from build123d import *

# Parameters (mm, degrees)
F0_W      = 120
F0_H      = 62
F1_DEPTH  = 1.5
F3_DEPTH  = 1.501
F5_DEPTH  = 1.501
F7_DEPTH  = 1.501
F8_R      = 1
F9_DEPTH  = 1.501
F10_W     = 7
F10_H     = 5
F11_DEPTH = 2
F13_DEPTH = 1
F14_W     = 3
F14_H     = 2.5
F15_DEPTH = 2
F16_W     = 3
F16_H     = 2.5
F17_DEPTH = 2
F18_W     = 3
F18_H     = 1
F19_DEPTH = 1
F20_W     = 4
F20_H     = 3
F21_DEPTH = 1
F23_DEPTH = 3
F24_W     = 1.5
F24_H     = 3
F25_DEPTH = 1
F26_W     = 5
F26_H     = 3.5
F27_DEPTH = 1.5
F28_W     = 3
F28_H     = 2
F29_DEPTH = 2
F30_W     = 3
F30_H     = 2
F31_DEPTH = 2
F32_R     = 2.5
F33_DEPTH = 2
F34_R     = 2.5
F35_DEPTH = 2
F36_W     = 3
F36_H     = 4
F37_DEPTH = 1
F38_W     = 2
F38_H     = 3
F39_DEPTH = 2


with BuildPart() as f1:
    # F0 (on Top) → F1 (new body)
    with BuildSketch(Plane.XY):
        with Locations((-17.615131, 6.410271)):
            Rectangle(F0_W, F0_H)
    extrude(amount=F1_DEPTH)

    # F2 (on face) → F3 (cut, through all)
    with BuildSketch(Plane.XY.offset(1.5)):
        with BuildLine():
            Line((-62.615131, -18.589729), (-62.615131, -24.589729))
            Line((-62.615131, -24.589729), (-34.615131, -24.589729))
            Line((-34.615131, -24.589729), (-34.615131, -18.589729))
            ThreePointArc((-34.615131, -18.589729), (-34.908024, -17.882622), (-35.615131, -17.589729))
            Line((-35.615131, -17.589729), (-61.615131, -17.589729))
            ThreePointArc((-61.615131, -17.589729), (-62.322238, -17.882622), (-62.615131, -18.589729))
        make_face()
    extrude(amount=-F3_DEPTH, mode=Mode.SUBTRACT)

    # F4 (on face) → F5 (cut, through all)
    with BuildSketch(Plane.XY.offset(1.5)):
        with BuildLine():
            Line((-20.615131, -17.589729), (-20.615131, -24.589729))
            Line((-20.615131, -24.589729), (-18.615131, -24.589729))
            Line((-18.615131, -24.589729), (-18.615131, -17.589729))
            ThreePointArc((-18.615131, -17.589729), (-19.615131, -16.589729), (-20.615131, -17.589729))
        make_face()
    extrude(amount=-F5_DEPTH, mode=Mode.SUBTRACT)

    # F6 (on face) → F7 (cut, through all)
    with BuildSketch(Plane.XY.offset(1.5)):
        with BuildLine():
            Line((22.384869, -17.543457), (22.384869, -24.589729))
            Line((22.384869, -24.589729), (24.384869, -24.589729))
            Line((24.384869, -24.589729), (24.384869, -17.543457))
            ThreePointArc((24.384869, -17.543457), (23.384869, -16.543457), (22.384869, -17.543457))
        make_face()
    extrude(amount=-F7_DEPTH, mode=Mode.SUBTRACT)

    # F8 (on face) → F9 (cut, through all)
    with BuildSketch(Plane.XY.offset(1.5)):
        with Locations((39.384869, -10.589729)):
            Circle(F8_R)
    extrude(amount=-F9_DEPTH, mode=Mode.SUBTRACT)

    # F10 (on face) → F11 (join)
    with BuildSketch(Plane.XY.offset(1.5)):
        with Locations((26.884869, -0.089729)):
            Rectangle(F10_W, F10_H)
    extrude(amount=F11_DEPTH)

    # F12 (on face) → F13 (join)
    with BuildSketch(Plane.XY.offset(1.5)):
        with BuildLine():
            Line((9.384869, 10.410271), (-2.615131, 10.410271))
            ThreePointArc((-2.615131, 10.410271), (-3.322238, 10.117378), (-3.615131, 9.410271))
            Line((-3.615131, 9.410271), (-3.615131, -8.589729))
            ThreePointArc((-3.615131, -8.589729), (-3.322238, -9.296836), (-2.615131, -9.589729))
            Line((-2.615131, -9.589729), (9.384869, -9.589729))
            ThreePointArc((9.384869, -9.589729), (10.091976, -9.296836), (10.384869, -8.589729))
            Line((10.384869, -8.589729), (10.384869, 9.410271))
            ThreePointArc((10.384869, 9.410271), (10.091976, 10.117378), (9.384869, 10.410271))
        make_face()
    extrude(amount=F13_DEPTH)

    # F14 (on face) → F15 (join)
    with BuildSketch(Plane.XY.offset(1.5)):
        with Locations((17.884869, 18.160271)):
            Rectangle(F14_W, F14_H)
    extrude(amount=F15_DEPTH)

    # F16 (on face) → F17 (join)
    with BuildSketch(Plane.XY.offset(1.5)):
        with Locations((17.884869, 23.660271)):
            Rectangle(F16_W, F16_H)
    extrude(amount=F17_DEPTH)

    # F18 (on face) → F19 (join)
    with BuildSketch(Plane.XY.offset(1.5)):
        with Locations((18.884869, 27.410271)):
            Rectangle(F18_W, F18_H)
    extrude(amount=F19_DEPTH)

    # F20 (on face) → F21 (join)
    with BuildSketch(Plane.XY.offset(1.5)):
        with Locations((17.384869, 30.910271)):
            Rectangle(F20_W, F20_H)
    extrude(amount=F21_DEPTH)

    # F22 (on face) → F23 (join)
    with BuildSketch(Plane.XY.offset(1.5)):
        with BuildLine():
            ThreePointArc((-14.115131, 21.910271), (-15.175791, 21.470931), (-15.615131, 20.410271))
            Line((-15.615131, 20.410271), (-15.615131, 13.910271))
            ThreePointArc((-15.615131, 13.910271), (-15.175791, 12.849611), (-14.115131, 12.410271))
            ThreePointArc((-14.115131, 12.410271), (-13.054471, 12.849611), (-12.615131, 13.910271))
            Line((-12.615131, 13.910271), (-12.615131, 20.410271))
            ThreePointArc((-12.615131, 20.410271), (-13.054471, 21.470931), (-14.115131, 21.910271))
        make_face()
    extrude(amount=F23_DEPTH)

    # F24 (on face) → F25 (join)
    with BuildSketch(Plane.XY.offset(1.5)):
        with Locations((-20.365131, 15.910271)):
            Rectangle(F24_W, F24_H)
    extrude(amount=F25_DEPTH)

    # F26 (on face) → F27 (join)
    with BuildSketch(Plane.XY.offset(1.5)):
        with Locations((-25.115131, 15.660271)):
            Rectangle(F26_W, F26_H)
    extrude(amount=F27_DEPTH)

    # F28 (on face) → F29 (join)
    with BuildSketch(Plane.XY.offset(1.5)):
        with Locations((-23.115131, 0.910271)):
            Rectangle(F28_W, F28_H)
    extrude(amount=F29_DEPTH)

    # F30 (on face) → F31 (join)
    with BuildSketch(Plane.XY.offset(1.5)):
        with Locations((-23.115131, -7.089729)):
            Rectangle(F30_W, F30_H)
    extrude(amount=F31_DEPTH)

    # F32 (on face) → F33 (join)
    with BuildSketch(Plane.XY.offset(1.5)):
        with Locations((-69.115131, 33.410271)):
            Circle(F32_R)
    extrude(amount=F33_DEPTH)

    # F34 (on face) → F35 (join)
    with BuildSketch(Plane.XY.offset(1.5)):
        with Locations((-69.115131, -20.716745)):
            Circle(F34_R)
    extrude(amount=F35_DEPTH)

    # F36 (on face) → F37 (join)
    with BuildSketch(Plane.XY.offset(1.5)):
        with Locations((-48.115131, 32.410271)):
            Rectangle(F36_W, F36_H)
    extrude(amount=F37_DEPTH)

    # F38 (on face) → F39 (join)
    with BuildSketch(Plane.XY.offset(1.5)):
        with Locations((-53.115131, 23.910271)):
            Rectangle(F38_W, F38_H)
    extrude(amount=F39_DEPTH)


solid = f1.part
Can you work these out from the model? Positions are in its coordinate system, mm. A direction names the side the tool comes from. Give positions to 0.01 mm unless a question says otherwise; leave off trailing zeros. Loops run counter-clockwise (first coordinate to the right, second up) from the corner with the lowest first, then second, coordinate; pieces in that order, holes last. Notation, with made-up numbers: (39.5, 58) - (78.5, 58) arc R19 cw to (78.5, 93) - close; hole circle Ø4 at (-22.5, -13). An arc over 180 degrees is marked (long way). Answer as a JSON object with one key per item and string values.
Q1. Imagine slicing it at C-C on x = 32. Write out the boundary of the cut face in (y, z), plus the area to 3 significant figures.
Geometry says:
{"outline": "(-24.59, 0) - (37.41, 0) - (37.41, 1.5) - (-24.59, 1.5) - close", "area": "93.0 mm²"}
Q2. Which directions (+Z, -Z, +X, -X, +Y, -Y) give clear straight access to the entire face, cutting with the end or side of a thin tool? Please do faces 1 (the flat face through (-25, 16, 3)), 2 (the cylindrical face through (-66.806, -21.674, 2.486)), 3 (the flat face through (-48, 32, 2.5)), 4 (the flat face through (17, 31, 2.5)), 5 (the flat face through (3, 1, 2.5)).
Geometry says:
{"face 1": "+Z, -X, +Y", "face 2": "+Z", "face 3": "+Z, +X, +Y, -Y", "face 4": "+Z, +X, +Y", "face 5": "+Z, +Y, -Y"}
Q3. If we mould it in two halves opening along Z, with no side actions, what happens to faces 6 (the flat face through (-69, 33, 3.5)), 7 (the cylindrical face through (-66.73, 34.16, 2.49)), 8 (the flat face through (-18, 7, 0))? For each: pulls with the +Z half, pulls with the -Z half, needs draft (parallel to the pull), parting line crosses it, or undercut.
Geometry says:
{"face 6": "pulls with the +Z half", "face 7": "needs draft", "face 8": "pulls with the -Z half"}
Q4. Imagine slicing it at A-A on y = 8. Write out the boundary of the cut face in (x, z), plus the area to 3 significant figures.
Geometry says:
{"outline": "(-77.62, 0) - (42.38, 0) - (42.38, 1.5) - (10.38, 1.5) - (10.38, 2.5) - (-3.62, 2.5) - (-3.62, 1.5) - (-77.62, 1.5) - close", "area": "194 mm²"}
Q5. Will these pins go through, and if not, where does the flat tip stop? P1, Ø2, axis at x = 18, y = 18.5, coming from the +Z side; P2, Ø0.6, axis at x = -22.5, z = 2.5, coming from the -Y side; P3, Ø1.1, axis at y = 32.5, z = 2, coming from the +X side; P4, Ø0.6, axis at y = 1, z = 2.5, coming from the -X side.
Geometry says:
{"P1": "z = 3.5", "P2": "y = -8.09", "P3": "x = 42.38", "P4": "x = -24.62"}
Q6. Imagine slicing it at B-B on x = -26.5. Write out the boundary of the cut face in (y, z).
Geometry says:
{"outline": "(-24.59, 0) - (37.41, 0) - (37.41, 1.5) - (17.41, 1.5) - (17.41, 3) - (13.91, 3) - (13.91, 1.5) - (-24.59, 1.5) - close"}
Q7. If I drill on L1, parallel to X at y = 1.5, z = 3; L2, parallel to Y at x = -25, z = 1.8; L3, parallel to X at y = -1.5, z = 2.3, over which ranges is the centre line in solid material (lowest first)?
Geometry says:
{"L1": "-24.62 to -21.62, 23.38 to 30.38", "L2": "13.91 to 17.41", "L3": "-3.62 to 10.38, 23.38 to 30.38"}
